```python
from build123d import *

# Parameters (mm, degrees)
BOSS_EXTRUDE1_DEPTH      = 120
BOSS_EXTRUDE2_DEPTH      = 120
SKETCH3_W                = 80
SKETCH3_H                = 80
BOSS_EXTRUDE3_DEPTH      = 40
BOSS_EXTRUDE4_DEPTH      = 40
BOSS_EXTRUDE5_DEPTH      = 120
SPLIT4_SURFACE_1_1_BACK  = 394.954
SPLIT4_SURFACE_1_1_DEPTH = 789.908
SPLIT4_SURFACE_1_2_BACK  = 394.954
SPLIT4_SURFACE_1_2_DEPTH = 789.908
SPLIT4_SURFACE_2_3_BACK  = 394.954
SPLIT4_SURFACE_2_3_DEPTH = 789.908
SPLIT4_SURFACE_2_4_BACK  = 394.954
SPLIT4_SURFACE_2_4_DEPTH = 789.908
CHAMFER4_SIZE            = 80


with BuildPart() as part:
    # Sketch1 → Boss-Extrude1 (new body)
    with BuildSketch(Plane.XY):
        Polygon((120, -100), (120, 20), (80, 20), (80, 100), (40, 100), (40, -60), (40, -100), align=None)
    extrude(amount=BOSS_EXTRUDE1_DEPTH)

    # Sketch1<3> → Boss-Extrude2 (add)
    with BuildSketch(Plane.XY):
        Polygon((120, -100), (120, 20), (80, 20), (80, 100), (40, 100), (40, -60), (40, -100), align=None)
    extrude(amount=-BOSS_EXTRUDE2_DEPTH)

    # Sketch3 → Boss-Extrude3 (add)
    with BuildSketch(Plane(origin=(80, 0, 0), x_dir=(0, 0, -1), z_dir=(1, 0, 0))):
        with Locations((80, 60)):
            Rectangle(SKETCH3_W, SKETCH3_H)
    extrude(amount=BOSS_EXTRUDE3_DEPTH)

    # Sketch1<4> → Boss-Extrude4 (add)
    with BuildSketch(Plane.XY):
        Polygon((40, -60), (40, 100), (-120, 100), (-120, -100), (-80, -100), (-80, -60), align=None)
    extrude(amount=BOSS_EXTRUDE4_DEPTH)

    # Sketch1<5> → Boss-Extrude5 (add)
    with BuildSketch(Plane.XY):
        Polygon((40, -60), (40, 100), (-120, 100), (-120, -100), (-80, -100), (-80, -60), align=None)
    extrude(amount=-BOSS_EXTRUDE5_DEPTH)


with BuildPart() as body_2:
    # Split4: the piece behind the surface
    add(part.part)
    # Split4 surface 1: a surface, the sketch's curves swept straight by 789.908 mm
    with BuildLine(Plane(origin=(0, 100, 0), x_dir=(1, 0, 0), z_dir=(0, 1, 0)).offset(-SPLIT4_SURFACE_1_1_BACK), mode=Mode.PRIVATE) as split4_surface_1_1_path:
        Line((-120, 0), (120, 0))
    split4_surface_1_1 = Shell.extrude(split4_surface_1_1_path.wire(), (0 * SPLIT4_SURFACE_1_1_DEPTH, 1 * SPLIT4_SURFACE_1_1_DEPTH, 0 * SPLIT4_SURFACE_1_1_DEPTH))
    split(bisect_by=split4_surface_1_1, keep=Keep.BOTTOM)


with BuildPart() as part_1:
    add(part.part)

    # Split4: split by a surface, the side it looks to stays
    # Split4 surface 1: a surface, the sketch's curves swept straight by 789.908 mm
    with BuildLine(Plane(origin=(0, 100, 0), x_dir=(1, 0, 0), z_dir=(0, 1, 0)).offset(-SPLIT4_SURFACE_1_2_BACK), mode=Mode.PRIVATE) as split4_surface_1_2_path:
        Line((-120, 0), (120, 0))
    split4_surface_1_2 = Shell.extrude(split4_surface_1_2_path.wire(), (0 * SPLIT4_SURFACE_1_2_DEPTH, 1 * SPLIT4_SURFACE_1_2_DEPTH, 0 * SPLIT4_SURFACE_1_2_DEPTH))
    split(bisect_by=split4_surface_1_2, keep=Keep.TOP)


with BuildPart() as body_3:
    # Split4 2: the piece behind the surface
    add(part_1.part)
    # Split4 surface 2: a surface, the sketch's curves swept straight by 789.908 mm
    with BuildLine(Plane(origin=(0, 100, 0), x_dir=(1, 0, 0), z_dir=(0, 1, 0)).offset(-SPLIT4_SURFACE_2_3_BACK), mode=Mode.PRIVATE) as split4_surface_2_3_path:
        Line((-120, 80), (120, 80))
    split4_surface_2_3 = Shell.extrude(split4_surface_2_3_path.wire(), (0 * SPLIT4_SURFACE_2_3_DEPTH, 1 * SPLIT4_SURFACE_2_3_DEPTH, 0 * SPLIT4_SURFACE_2_3_DEPTH))
    split(bisect_by=split4_surface_2_3, keep=Keep.BOTTOM)

    # Chamfer4
    chamfer4_edges = [body_3.edges().sort_by_distance(p)[0] for p in [
        (-120, 100, -40),
    ]]
    chamfer(chamfer4_edges, length=CHAMFER4_SIZE)


with BuildPart() as part_2:
    add(part_1.part)

    # Split4 2: split by a surface, the side it looks to stays
    # Split4 surface 2: a surface, the sketch's curves swept straight by 789.908 mm
    with BuildLine(Plane(origin=(0, 100, 0), x_dir=(1, 0, 0), z_dir=(0, 1, 0)).offset(-SPLIT4_SURFACE_2_4_BACK), mode=Mode.PRIVATE) as split4_surface_2_4_path:
        Line((-120, 80), (120, 80))
    split4_surface_2_4 = Shell.extrude(split4_surface_2_4_path.wire(), (0 * SPLIT4_SURFACE_2_4_DEPTH, 1 * SPLIT4_SURFACE_2_4_DEPTH, 0 * SPLIT4_SURFACE_2_4_DEPTH))
    split(bisect_by=split4_surface_2_4, keep=Keep.TOP)


with BuildPart() as body_3_1:
    add(body_3.part)

    # Combine2: union part, body 2
    add(part_2.part)
    add(body_2.part)


solid = body_3_1.part
```
Check sheet for the modelled part. Datum: model origin and axes. Units: mm. A direction names the side the tool comes from. Give positions to 0.01 mm unless a question says otherwise; leave off trailing zeros. Loops run counter-clockwise (first coordinate to the right, second up) from the corner with the lowest first, then second, coordinate; pieces in that order, holes last. Notation, with made-up numbers: M 69,81.5 L 79,81.5 A17 ccw 79,99.5 Z; hole C 61.25,38.5 d7. An arc over 180 degrees is marked long. Answer in a Markdown table with one row per item.
1) Cross-section at D-D (y = -23.5). Enter the section's corners in (x, z).
Solutions:
| item | result |
|---|---|
| outline | M -120,-120 L 120,-120 L 120,120 L 40,120 L 40,40 L -120,40 Z |
2) Cross-section at B-B (x = -84). Enter the section's corners in (y, z), plus the area to 3 significant figures.
Solutions:
| item | result |
|---|---|
| outline | M -100,-120 L 100,-120 L 100,-80 L 56,-80 L 56,0 L 100,0 L 100,40 L -100,40 Z |
| area | 28,500 mm^2 |
3) Cross-section at C-C (z = -16.5). Enter the section's corners in (x, y), plus the area to 3 significant figures.
Solutions:
| item | result |
|---|---|
| outline | M -120,-100 L -80,-100 L -80,-60 L 40,-60 L 40,-100 L 120,-100 L 120,20 L 80,20 L 80,100 L -40,100 L -120,20 Z |
| area | 36,800 mm^2 |
4) Thickness scan on line 1 (X direction, y = -72.5, z = -103); line 2 (X direction, y = 39, z = 46.5); line 3 (Z direction, x = -63, y = -10). Record the ranges inside material, lowest first.
Solutions:
| item | result |
|---|---|
| line 1 | x = -120 to -80, 40 to 120 |
| line 2 | x = 40 to 80 |
| line 3 | z = -120 to 40 |
5) Depth check by flat-ended pin: pin 1 (5 mm diameter, centred on y = 30, z = 5, fed in from +X); pin 2 (20 mm diameter, centred on x = 93, y = 67.5, fed in from +Z); pin 3 (2 mm diameter, centred on x = 11.5, z = -72, fed in from -Y). Enter the tip coordinate at first touch or a pass-through.
Solutions:
| item | result |
|---|---|
| pin 1 | stops at x = 80 |
| pin 2 | stops at z = -40 |
| pin 3 | stops at y = -60 |
6) Mould release check, pull along Z, two halves, no side actions. Record for faces 5 (the face through (-81, 59, -41)), 6 (the face through (120, -21, -25)), 7 (the face through (-41, 24, 40)): released by +Z, released by -Z, zero draft, split by the parting line, or undercut.
Solutions:
| item | result |
|---|---|
| face 5 | undercut |
| face 6 | zero draft |
| face 7 | released by +Z |
7) Tool access check on faces 1 (the face through (-80, -80, -39)), 2 (the face through (40, -21, 55)), 3 (the face through (-98, 77, -80)), 4 (the face through (100, 20, 41)). Record the directions out of +Z, -Z, +X, -X, +Y, -Y that give a thin tool (end or side, any length) a straight path to the whole face; none if there is none.
Solutions:
| item | result |
|---|---|
| face 1 | +Z, -Z, -Y |
| face 2 | +Z, -Y |
| face 3 | -X, +Y |
| face 4 | +Z, +X, +Y |
8) Cross-section at A-A (y = -71). Enter the section's corners in (x, z), plus the area to 3 significant figures.
Solutions:
| item | result |
|---|---|
| outline | M -120,-120 L -80,-120 L -80,40 L -120,40 Z; M 40,-120 L 120,-120 L 120,120 L 40,120 Z |
| area | 25,600 mm^2 |
